```python
from build123d import *

# Parameters (mm, degrees)
GEARBOX_DEPTH                            = 9
AXLE_MOUNT_HOLE_BASE_SKETCH_R            = 0.8
SCREW_HOLES_DEPTH                        = 0.8
SCREW_ROOM_BASE_W                        = 3
SCREW_ROOM_BASE_H                        = 3
SCREW_ROOM_DEPTH                         = 2
AXLE_MOUNT_HOLE_BASE_SKETCH_3_R          = 2
AXLE_BASE_DEPTH                          = 0.7
SKETCH4_R                                = 1.5
AXLE_NON_NOTCHED_DEPTH                   = 0.3
AXLE_NOTCHED_DEPTH                       = 9
MOTOR_DEPTH                              = 15.4
REAR_AXLE_BEARING_TERMINAL_BASE_SKETCH_R = 2.5
REAR_AXLE_BEARING_DEPTH                  = 0.8
REAR_AXLE_BEARING_TERMINAL_BASE_SK_2_W   = 0.4
REAR_AXLE_BEARING_TERMINAL_BASE_SK_2_H   = 2
TERMINALS_DEPTH                          = 1.8


with BuildPart() as part:
    # Gearbox base sketch → Gearbox (new body)
    with BuildSketch(Plane(origin=(0, 0, 0), x_dir=(1, 0, 0), z_dir=(0, 1, 0))):
        with BuildLine():
            Line((-4.992296279, 5), (4.992296279, 5))
            ThreePointArc((4.992296279, 5), (5.704850414, 4.704850414), (6, 3.992296279))
            Line((6, 3.992296279), (6, -3.992296279))
            ThreePointArc((6, -3.992296279), (5.704850414, -4.704850414), (4.992296279, -5))
            Line((4.992296279, -5), (-4.992296279, -5))
            ThreePointArc((-4.992296279, -5), (-5.704850414, -4.704850414), (-6, -3.992296279))
            Line((-6, -3.992296279), (-6, 3.992296279))
            ThreePointArc((-6, 3.992296279), (-5.704850414, 4.704850414), (-4.992296279, 5))
        make_face()
    extrude(amount=GEARBOX_DEPTH)

    # Axle _ mount hole base sketch → Screw holes (cut)
    with BuildSketch(Plane(origin=(0, 9, 0), x_dir=(1, 0, 0), z_dir=(0, 1, 0))):
        with Locations(Location((-4.5, 0, 0), (0, 0, 270))):
            Circle(AXLE_MOUNT_HOLE_BASE_SKETCH_R)
        with Locations(Location((4.5, 0, 0), (0, 0, 270))):
            Circle(AXLE_MOUNT_HOLE_BASE_SKETCH_R)
    extrude(amount=-SCREW_HOLES_DEPTH, mode=Mode.SUBTRACT)

    # Screw room base → Screw room (cut)
    with BuildSketch(Plane(origin=(0, 8.2, 0), x_dir=(1, 0, 0), z_dir=(0, 1, 0))):
        with Locations((-4.5, 0)):
            Rectangle(SCREW_ROOM_BASE_W, SCREW_ROOM_BASE_H)
        with Locations((4.5, 0)):
            Rectangle(SCREW_ROOM_BASE_W, SCREW_ROOM_BASE_H)
    extrude(amount=-SCREW_ROOM_DEPTH, mode=Mode.SUBTRACT)

    # Axle _ mount hole base sketch_3 → Axle base (add)
    with BuildSketch(Plane(origin=(0, 9, 0), x_dir=(1, 0, 0), z_dir=(0, 1, 0))):
        with Locations(Location((0, 0, 0), (0, 0, 270))):
            Circle(AXLE_MOUNT_HOLE_BASE_SKETCH_3_R)
    extrude(amount=AXLE_BASE_DEPTH)

    # Sketch4 → Axle non-notched (add)
    with BuildSketch(Plane(origin=(0, 9.7, 0), x_dir=(1, 0, 0), z_dir=(0, 1, 0))):
        with Locations(Location((0, 0, 0), (0, 0, 270))):
            Circle(SKETCH4_R)
    extrude(amount=AXLE_NON_NOTCHED_DEPTH)

    # Axle notched base sketch → Axle notched (add)
    with BuildSketch(Plane(origin=(0, 10, 0), x_dir=(1, 0, 0), z_dir=(0, 1, 0))):
        with BuildLine():
            Line((1.118033989, 1), (-1.118033989, 1))
            ThreePointArc((-1.118033989, 1), (-0.535233135, -1.401258538), (1.5, 0))
            ThreePointArc((1.5, 0), (1.401258538, 0.535233135), (1.118033989, 1))
        make_face()
    extrude(amount=AXLE_NOTCHED_DEPTH)

    # Motor base sketch → Motor (add)
    with BuildSketch(Plane.XZ):
        with BuildLine():
            ThreePointArc((6, 0.776208735), (5.155527224, 3.165918356), (3.406244266, 5))
            Line((3.406244266, 5), (-3.406244266, 5))
            ThreePointArc((-3.406244266, 5), (-5.155527224, 3.165918356), (-6, 0.776208735))
            Line((-6, 0.776208735), (-6, -0.776208735))
            ThreePointArc((-6, -0.776208735), (-5.155527224, -3.165918356), (-3.406244266, -5))
            Line((-3.406244266, -5), (3.406244266, -5))
            ThreePointArc((3.406244266, -5), (5.155527224, -3.165918356), (6, -0.776208735))
            Line((6, -0.776208735), (6, 0.776208735))
        make_face()
        with BuildLine():
            Line((-6, -0.776208735), (-6, 0.776208735))
            ThreePointArc((-6, 0.776208735), (-6.05, 0), (-6, -0.776208735))
        make_face()
        with BuildLine():
            ThreePointArc((3.33166625, -5.05), (3.369048015, -5.025138353), (3.406244266, -5))
            Line((3.406244266, -5), (-3.406244266, -5))
            ThreePointArc((-3.406244266, -5), (-3.369048015, -5.025138353), (-3.33166625, -5.05))
            Line((-3.33166625, -5.05), (3.33166625, -5.05))
        make_face()
        with BuildLine():
            ThreePointArc((3.406244266, 5), (3.369048015, 5.025138353), (3.33166625, 5.05))
            Line((3.33166625, 5.05), (-3.33166625, 5.05))
            ThreePointArc((-3.33166625, 5.05), (-3.369048015, 5.025138353), (-3.406244266, 5))
            Line((-3.406244266, 5), (3.406244266, 5))
        make_face()
        with BuildLine():
            ThreePointArc((6.05, 0), (6.03748706, 0.38890873), (6, 0.776208735))
            Line((6, 0.776208735), (6, -0.776208735))
            ThreePointArc((6, -0.776208735), (6.03748706, -0.38890873), (6.05, 0))
        make_face()
    extrude(amount=MOTOR_DEPTH)

    # Rear axle bearing _ terminal base sketch → Rear axle bearing (add)
    with BuildSketch(Plane.XZ.offset(15.4)):
        with Locations(Location((0, 0, 0), (0, 0, 270))):
            Circle(REAR_AXLE_BEARING_TERMINAL_BASE_SKETCH_R)
    extrude(amount=REAR_AXLE_BEARING_DEPTH)

    # Rear axle bearing _ terminal base sk 2 → Terminals (add)
    with BuildSketch(Plane.XZ.offset(15.4)):
        with Locations((-3.1, 0)):
            Rectangle(REAR_AXLE_BEARING_TERMINAL_BASE_SK_2_W, REAR_AXLE_BEARING_TERMINAL_BASE_SK_2_H)
        with Locations((3.1, 0)):
            Rectangle(REAR_AXLE_BEARING_TERMINAL_BASE_SK_2_W, REAR_AXLE_BEARING_TERMINAL_BASE_SK_2_H)
    extrude(amount=TERMINALS_DEPTH)


solid = part.part
```
Model file for the job. Use its own axes, mm. A direction names the side the tool comes from. Coordinates: 2 decimals unless noted, no trailing zeros. Write each loop counter-clockwise with the first axis right and the second up, starting at its lowest first coordinate (ties: lowest second). Pieces come first, ordered by that corner, then holes. Notation, with made-up numbers: (-37, 4) - (-16, 4) arc R33 cw to (-16, 40) - close; hole circle Ø10 at (-5.75, -2). An arc over 180 degrees is marked (long way). One line per item, written item: value. Start each with the question number.
1. Mould opens along Z. For faces 6 (the flat face through (-3, 7, 0)), 7 (the cylindrical face through (5.71, 4.44, 4.7)), 8 (the flat face through (-4, 8.2, -1)), 9 (the flat face through (6, 4, 0)) say: released by +Z, released by -Z, zero draft, split by the parting line, or undercut.
2. Slice it at B-B (z = -3.25). Write the cut outline in (x, y).
3. Slice it at C-C (x = 0). Write the cut outline in (y, z).
4. Probe line 1 (X direction, y = 8.8, z = 0); line 2 (Y direction, x = 1.5, z = 4.25); line 3 (Z direction, x = 4.25, y = 6.5). List the from-to ranges inside material, lowest first. Write a range as from..to.
5. Tool access for faces 1 (the flat face through (5, 0, -4)), 2 (the cylindrical face through (-5.28, 8.61, -0.17)), 3 (the flat face through (5, 8.2, -1)), 4 (the flat face through (0, 4, -5)), 5 (the flat face through (-5, 6.2, 0)): list every direction of +Z, -Z, +X, -X, +Y, -Y with a clear straight run to the whole face (end or side of a thin tool).
6. Slice it at D-D (y = 17). Write the cut outline in (x, z), plus the area to 3 significant figures.
7. Slice it at A-A (y = 7). Write the cut outline in (x, z), plus the area to 3 significant figures.
8. Flat gauge pins, fed straight in: pin 1 (1.6 mm diameter, centred on x = 4.5, y = 7.5, fed in from -Z); pin 2 (2 mm diameter, centred on y = 6, z = 0.5, fed in from -X); pin 3 (2.5 mm diameter, centred on x = 4.5, z = 0.5, fed in from +Y); pin 4 (5 mm diameter, centred on x = -1.5, z = 1.5, fed in from -Y). Where does each tip first touch, or does it go through?
Answers below:
1. face 6: undercut
1. face 7: released by +Z
1. face 8: undercut
1. face 9: zero draft
2. outline: (-6, 0) - (-5.1, 0) - (-5.1, -15.4) - (5.1, -15.4) - (5.1, 0) - (6, 0) - (6, 9) - (-6, 9) - close
3. outline: (-16.2, -2.5) - (-15.4, -2.5) - (-15.4, -5.05) - (0, -5.05) - (0, -5) - (9, -5) - (9, -2) - (9.7, -2) - (9.7, -1.5) - (10, -1.5) - (10, -1) - (19, -1) - (19, 1.5) - (9.7, 1.5) - (9.7, 2) - (9, 2) - (9, 5) - (0, 5) - (0, 5.05) - (-15.4, 5.05) - (-15.4, 2.5) - (-16.2, 2.5) - close
4. line 1: x = -6..-5.3, -3.7..3.7, 5.3..6
4. line 2: y = -15.4..9
4. line 3: z = -5..-1.5, 1.5..5
5. face 1: -Z, +X, -Y
5. face 2: +Y
5. face 3: +X
5. face 4: -Z, +X, -X, +Y
5. face 5: -X
6. outline: (-1.12, -1) - (1.12, -1) arc R1.5 ccw (long way) to start
6. area: 6.29 mm^2
7. outline: (-6, -3.99) arc R1.01 ccw to (-4.99, -5) - (4.99, -5) arc R1.01 ccw to (6, -3.99) - (6, -1.5) - (3, -1.5) - (3, 1.5) - (6, 1.5) - (6, 3.99) arc R1.01 ccw to (4.99, 5) - (-4.99, 5) arc R1.01 ccw to (-6, 3.99) - (-6, 1.5) - (-3, 1.5) - (-3, -1.5) - (-6, -1.5) - close
7. area: 101 mm^2
8. pin 1: stops at z = -5
8. pin 2: stops at x = -6
8. pin 3: stops at y = 9
8. pin 4: stops at y = -17.2
